Build history of the part. All positions in model axes, mm. Face numbers are marked on the shaded views. Round coordinates to 2 decimals unless told otherwise and drop trailing zeros. Order: outer loops, then holes, each group sorted by start corner. A loop starts at its lowest first (then second) coordinate and runs counter-clockwise, first axis right, second up. Notation, with made-up numbers: (75, 20) -> (80, 20) arc R18 ccw to (80, 45) -> close; hole circle Ø6 at (33.5, 32.5). An arc over 180 degrees is marked (long way). Write item = value, one per line.
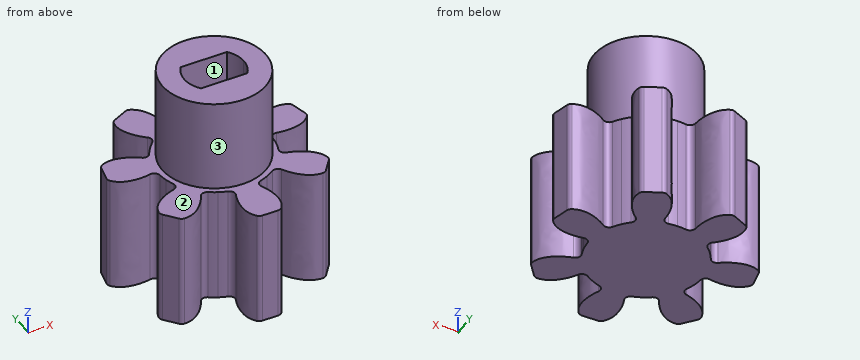
from build123d import *

# Parameters (mm, degrees)
F1_DEPTH = 10
F2_COUNT = 7
F2_ANGLE = 308.5714285714
F3_R     = 4.5
F4_DEPTH = 8


with BuildPart() as f1:
    # F0 (on Top) → F1 (new body)
    with BuildSketch(Plane.XY):
        with BuildLine():
            Line((2.1694186956, -4.5048443395), (0, 0))
            Line((0, 0), (-2.1694186956, -4.5048443395))
            ThreePointArc((-2.1694186956, -4.5048443395), (-1.8131769027, -4.6596555151), (-1.4459926079, -4.7863457228))
            ThreePointArc((-1.4459926079, -4.7863457228), (-1.1360019143, -5.0567785338), (-1.1337288621, -5.4681457281))
            add(Edge.make_bspline(
                [(-1.0826978963, -8.6677274808), (-1.4220303963, -8.2489427131), (-1.6630910077, -7.2785752045), (-1.3914458364, -6.0476801005), (-1.1337288621, -5.4681457281)],
                knots=[0.0602672768, 0.0602672768, 0.0602672768, 0.0602672768, 0.4600969779, 0.8689019138, 0.8689019138, 0.8689019138, 0.8689019138], degree=3))
            ThreePointArc((-1.0826978963, -8.6677274808), (-0.9094070817, -8.8042759726), (-0.6942189728, -8.8529511696))
            Line((-0.6942189728, -8.8529511696), (0.6942189728, -8.8529511696))
            ThreePointArc((0.6942189728, -8.8529511696), (0.9094070817, -8.8042759726), (1.0826978963, -8.6677274808))
            add(Edge.make_bspline(
                [(1.0826978963, -8.6677274808), (1.4220303963, -8.2489427131), (1.6630910077, -7.2785752045), (1.3914458364, -6.0476801005), (1.1337288621, -5.4681457281)],
                knots=[0.0602672768, 0.0602672768, 0.0602672768, 0.0602672768, 0.4600969779, 0.8689019138, 0.8689019138, 0.8689019138, 0.8689019138], degree=3))
            ThreePointArc((1.1337288621, -5.4681457281), (1.1360019143, -5.0567785338), (1.4459926079, -4.7863457228))
            ThreePointArc((1.4459926079, -4.7863457228), (1.8131769027, -4.6596555151), (2.1694186956, -4.5048443395))
        make_face()
    extrude(amount=F1_DEPTH)

    # F2: F1 ×7 about axis
    f2_axis = Axis((0, 0, 5), (0, 0, -1))


with BuildPart() as f1_1:
    add(f1.part)
    for i in range(1, F2_COUNT):
        add(f1.part.rotate(f2_axis, i * F2_ANGLE / (F2_COUNT - 1)))

    # F3 (on face) → F4 (join)
    with BuildSketch(Plane.XY.offset(10)):
        Circle(F3_R)
        with BuildLine():
            ThreePointArc((2.0493901532, 1.6), (2.458496939, 0.8460453894), (2.6, 0))
            ThreePointArc((2.6, 0), (2.458496939, -0.8460453894), (2.0493901532, -1.6))
            ThreePointArc((2.0493901532, -1.6), (0, -2.6), (-2.0493901532, -1.6))
            ThreePointArc((-2.0493901532, -1.6), (-2.6, 0), (-2.0493901532, 1.6))
            ThreePointArc((-2.0493901532, 1.6), (0, 2.6), (2.0493901532, 1.6))
        make_face(mode=Mode.SUBTRACT)
        with BuildLine():
            Line((-2.0493901532, 1.6), (2.0493901532, 1.6))
            ThreePointArc((2.0493901532, 1.6), (0, 2.6), (-2.0493901532, 1.6))
        make_face()
        with BuildLine():
            ThreePointArc((-2.0493901532, -1.6), (0, -2.6), (2.0493901532, -1.6))
            Line((2.0493901532, -1.6), (-2.0493901532, -1.6))
        make_face()
    extrude(amount=F4_DEPTH)


solid = f1_1.part
Q1. Cut at B-B, the plane x = 0.25. List the corners of the cut face in (y, z), and give its area (3 significant figures).
Check values:
outline = (-8.85, 0) -> (4.99, 0) -> (4.99, 10) -> (4.49, 10) -> (4.49, 18) -> (1.6, 18) -> (1.6, 10) -> (-1.6, 10) -> (-1.6, 18) -> (-4.49, 18) -> (-4.49, 10) -> (-8.85, 10) -> close
area = 185 mm²
Q2. Flat gauge pins, fed straight in: pin 1 (1.5 mm diameter, centred on x = -1.5, z = 12, fed in from -Y); pin 2 (4.5 mm diameter, centred on x = 1, z = 13, fed in from +Y); pin 3 (3.5 mm diameter, centred on x = -0.5, z = 15.5, fed in from -Y); pin 4 (3 mm diameter, centred on y = -6.5, z = 14, fed in from +X). Where does each tip first touch, or does it go through?
Check values:
pin_1 = -4.44
pin_2 = 4.5
pin_3 = -4.5
pin_4 = through
Q3. Mould opens along Y. For the marked faces 1, 2 and 3 say: released by +Y, released by -Y, zero draft, split by the parting line, or undercut.
Check values:
face_1 = undercut
face_2 = zero draft
face_3 = split by the parting line
Q4. Probe probe 1 along Y at (x, z) = (0.5, 14.75); probe 2 along Z at (x, y) = (4.75, 1.5); probe 3 along X at (y, z) = (3.5, 5.5). List the from-to ranges inside material, lowest first.
Check values:
probe_1 = -4.47 to -1.6, 1.6 to 4.47
probe_2 = 0 to 10
probe_3 = -3.57 to 3.57
Q5. Cut at A-A, the plane z = 11.25. List the corners of the cut face in (x, y).
Check values:
outline = circle Ø9 at (0, 0); hole (-2.05, -1.6) -> (2.05, -1.6) arc R2.6 ccw to (2.05, 1.6) -> (-2.05, 1.6) arc R2.6 ccw to start
